Geometry: final body of the model. Coordinates: model frame, mm. A direction names the side the tool comes from. Coordinates: 2 decimals unless noted, no trailing zeros. Write each loop counter-clockwise with the first axis right and the second up, starting at its lowest first coordinate (ties: lowest second). Pieces come first, ordered by that corner, then holes.
from build123d import *

# Parameters (mm, degrees)
SKETCH_R           = 23.7
PAD_DEPTH          = 1
POCKET_DEPTH       = 135.083363
POLARPATTERN_COUNT = 12
SKETCH002_R        = 23.7
SKETCH002_R_2      = 22.7
PAD001_DEPTH       = 5
SKETCH003_R        = 22.7
SKETCH003_R_2      = 21.7
PAD002_DEPTH       = 2
SKETCH004_R        = 3
POCKET001_DEPTH    = 5.001


with BuildPart() as part:
    # Sketch → Pad (new body)
    with BuildSketch(Plane.XY):
        Circle(SKETCH_R)
    extrude(amount=PAD_DEPTH)

    # Sketch001 → Pocket (cut, through all)
    with BuildSketch(Plane.XY):
        with BuildLine():
            ThreePointArc((-0.5, 4.941518), (0, 4.496592), (0.5, 4.941518))
            Line((2.000001, 17.766074), (0.5, 4.941518))
            ThreePointArc((2.000001, 17.766074), (-7e-06, 20.013635), (-1.999999, 17.766059))
            Line((-0.5, 4.941518), (-1.999999, 17.766059))
        make_face()
    pocket = extrude(amount=POCKET_DEPTH, mode=Mode.SUBTRACT)

    # PolarPattern: Pocket ×12 about axis
    polarpattern_axis = Axis((0, 0, 0), (0, 0, 1))
    for i in range(1, POLARPATTERN_COUNT):
        add(pocket.rotate(polarpattern_axis, i * 360 / POLARPATTERN_COUNT), mode=Mode.SUBTRACT)

    # Sketch002 → Pad001 (join)
    with BuildSketch(Plane.XY):
        Circle(SKETCH002_R)
        Circle(SKETCH002_R_2, mode=Mode.SUBTRACT)
    extrude(amount=PAD001_DEPTH)

    # Sketch003 → Pad002 (join)
    with BuildSketch(Plane.XY):
        Circle(SKETCH003_R)
        Circle(SKETCH003_R_2, mode=Mode.SUBTRACT)
    extrude(amount=PAD002_DEPTH)

    # Sketch004 → Pocket001 (cut, through all)
    with BuildSketch(Plane.XY):
        Circle(SKETCH004_R)
    extrude(amount=POCKET001_DEPTH, mode=Mode.SUBTRACT)


solid = part.part
Item 1: Section B-B, the plane y = 18.5. Output: boundary loops of the cut face in (x, z), plus the area to 3 significant figures.
Derived:
outline: (-14.81, 0) - (-1.95, 0) - (-1.95, 1) - (-11.34, 1) - (-11.34, 2) - (-13.15, 2) - (-13.15, 5) - (-14.81, 5) - close; (1.95, 0) - (14.81, 0) - (14.81, 5) - (13.15, 5) - (13.15, 2) - (11.34, 2) - (11.34, 1) - (1.95, 1) - close
area: 42.6 mm2
Item 2: Pin query (flat end, axial travel): pin 1 (1 mm diameter, centred on y = -8, z = 3.5, fed in from -X); pin 2 (2.5 mm diameter, centred on x = 18, y = 0, fed in from +Z); pin 3 (5 mm diameter, centred on x = 9, y = 15.59, fed in from -Z); pin 4 (2 mm diameter, centred on x = 11, z = 0.5, fed in from +Y). Return the tip coordinate at first contact, or that it passes through.
Derived:
pin 1: stops at x = -22.48
pin 2: passes through
pin 3: stops at z = 0
pin 4: stops at y = 21.49
Item 3: Material intervals for probe 1 along X at (y, z) = (9, 0.45); probe 2 along X at (y, z) = (-16, 0.35); probe 3 along Z at (x, y) = (21.5, 4), sorted ascending.
Derived:
probe 1: x = -21.92 to -17.6, -12.22 to -6.6, -3.97 to -0.97, 0.97 to 3.97, 6.6 to 12.22, 17.6 to 21.92
probe 2: x = -17.48 to -10.97, -6.98 to -1.79, 1.79 to 6.98, 10.97 to 17.48
probe 3: z = 0 to 2
Item 4: Section A-A, the plane x = -9. State how many separate pieces and enclosed holes the cut face has, plus the area to 3 significant figures.
Derived:
separate pieces: 6
enclosed holes: 0
area: 36.7 mm2
Item 5: Pull-direction query (Y, two-part tool) for faces 4 (the flat face through (11.26, 1.24, 0.49)), 5 (the flat face through (0, -23, 5)), 6 (the flat face through (4.559, 10.375, 0.493)); classes: released by +Y, released by -Y, zero draft, split by the parting line, or undercut.
Derived:
face 4: undercut
face 5: zero draft
face 6: undercut
Item 6: Set-up query: faces 1 (the flat face through (-11.44, 1.26, 0.49)), 2 (the flat face through (5, -5, 0)), 3 (the flat face through (5, -5, 1)). Return all of +Z, -Z, +X, -X, +Y, -Y with unobstructed straight access to the full face (end or side cutting, diameter ignored); none if empty.
Derived:
face 1: +Z, -Z
face 2: -Z, +X, -X, +Y, -Y
face 3: +Z
Item 7: Section D-D, the plane z = 3.2. Output: boundary loops of the cut face in (x, y).
Derived:
outline: circle Ø47.4 at (0, 0); hole circle Ø45.4 at (0, 0)
Item 8: Section C-C, the plane x = 12. Output: boundary loops of the cut face in (y, z), plus the area to 3 significant figures.
Derived:
outline: (-20.44, 0) - (-8.84, 0) - (-8.84, 1) - (-18.08, 1) - (-18.08, 2) - (-19.27, 2) - (-19.27, 5) - (-20.44, 5) - close; (-5.26, 0) - (-1.33, 0) - (-1.33, 1) - (-5.26, 1) - close; (1.33, 0) - (5.26, 0) - (5.26, 1) - (1.33, 1) - close; (8.84, 0) - (20.44, 0) - (20.44, 5) - (19.27, 5) - (19.27, 2) - (18.08, 2) - (18.08, 1) - (8.84, 1) - close
area: 42.8 mm2
